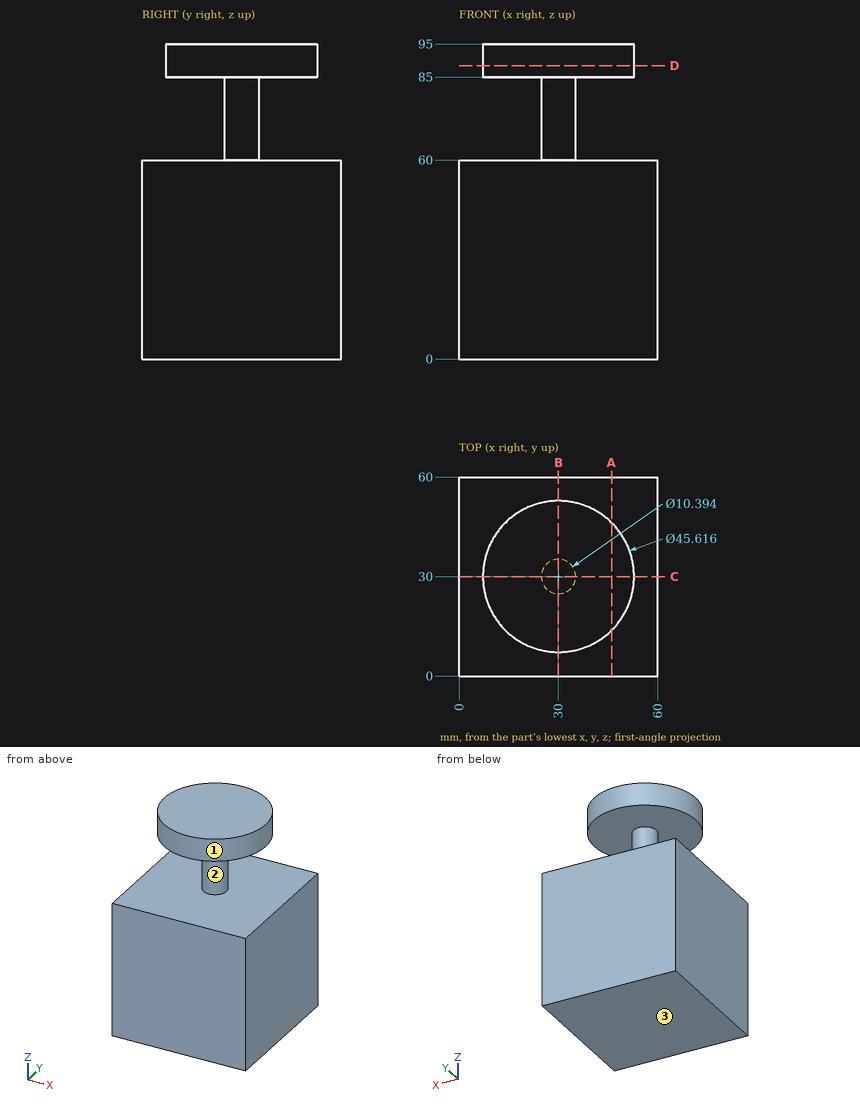
Study the drawing (mm; zero at the part's minimum x, y, z) and answer. Coordinates: 2 decimals unless noted, no trailing zeros. Write each loop counter-clockwise with the first axis right and the second up, starting at its lowest first coordinate (ties: lowest second). Pieces come first, ordered by that corner, then holes. Notation, with made-up numbers: (23.5, -6.5) - (47.5, -6.5) arc R18 ccw to (47.5, 19.5) - close; hole circle Ø3 at (-28, -38). An arc over 180 degrees is marked (long way). Answer as a JSON object with one key per item and string values.
Q1. Find section A-A (x = 46). Write down the section's boundary in (y, z) (1 decimal), plus the area to 4 significant figures.
Results list:
{"outline": "(0, 0) - (60, 0) - (60, 60) - (0, 60) - close; (13.7, 85) - (46.3, 85) - (46.3, 95) - (13.7, 95) - close", "area": "3,925 mm^2"}
Q2. Find section D-D (z = 88.5). Write down the section's boundary in (x, y), plus the area to 3 significant figures.
Results list:
{"outline": "circle Ø45.62 at (30, 30)", "area": "1,630 mm^2"}
Q3. For a pull along Z with two mould halves and no side action, classify the marked faces 1, 2 and 3 as pulls with the +Z half, pulls with the -Z half, needs draft (parallel to the pull), parting line crosses it, or undercut.
Results list:
{"face 1": "needs draft", "face 2": "undercut", "face 3": "pulls with the -Z half"}
Q4. Find section B-B (x = 30). Write down the section's boundary in (y, z), plus the area to 3 significant figures.
Results list:
{"outline": "(0, 0) - (60, 0) - (60, 60) - (35.2, 60) - (35.2, 85) - (52.81, 85) - (52.81, 95) - (7.19, 95) - (7.19, 85) - (24.8, 85) - (24.8, 60) - (0, 60) - close", "area": "4,320 mm^2"}
Q5. Consider L1, parallel to Z at x = 18.5, y = 47; L2, parallel to Z at x = 21.5, y = 57.5; L3, parallel to X at y = 20, z = 88.5. Determine where each line is inside the solid, lowest interval first. Write a range as from..to.
Results list:
{"L1": "z = 0..60, 85..95", "L2": "z = 0..60", "L3": "x = 9.5..50.5"}
